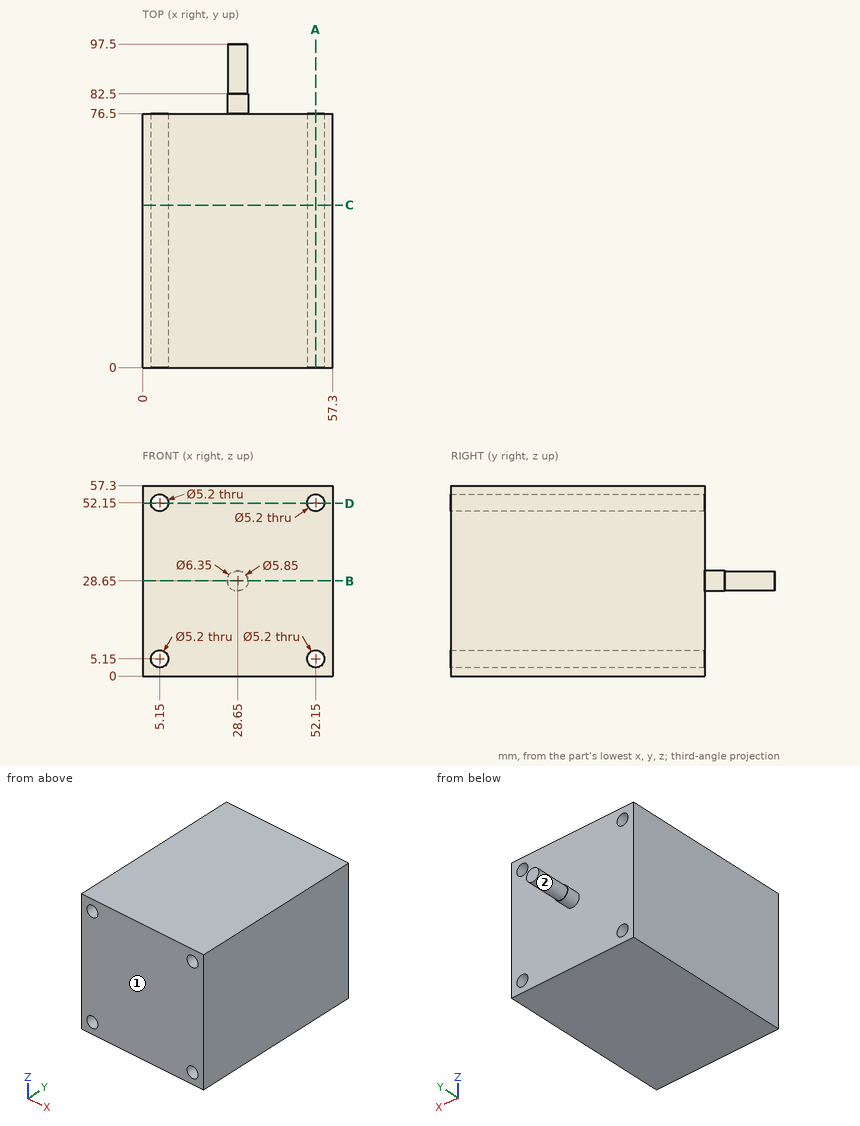
The figure shows three views and two pictorial views of one solid part (mm, origin at its lowest corner). Answer the questions. A direction names the side the tool comes from. Coordinates: 2 decimals unless noted, no trailing zeros. Loops run counter-clockwise (first coordinate to the right, second up) from the corner with the lowest first, then second, coordinate; pieces in that order, holes last. Notation, with made-up numbers: M -36.5,23 L -15.5,23 A10 ccw -15.5,40 Z; hole C 75.25,58.5 d11. An arc over 180 degrees is marked long. Answer as CSV lines item,"result". Start each with the question number.
(1) The part is cut by section D-D (z = 52). Give the vertices of the cut face in (x, y), and give its area (3 significant figures).
(2) The part is cut by section A-A (x = 52.15). Give the vertices of the cut face in (y, z).
(3) The part is cut by section B-B (z = 28.65). Give the vertices of the cut face in (x, y) (3 decimals).
(4) The part is cut by section C-C (y = 49). Give the vertices of the cut face in (x, z), and give its area (3 significant figures).
(5) Find the intervals of material crossed by L1, parallel to X at y = 51.5, z = 52.15; L2, parallel to Z at x = 4, y = 72, in increasing order. Write a range as [from, to].
(6) For the marked faces 1 and 2, determine the directions among +Z, -Z, +X, -X, +Y, -Y from which every point of the face is accessible in a straight line to the end or side of a thin tool.
(7) Given pin 1 (5 mm diameter, centred on x = 17, z = 17, fed in from -Y); pin 2 (4 mm diameter, centred on x = 33, z = 21.5, fed in from +Y), each flat-ended and moving along its own axis, determine where each tip first touches the part or whether it passes through.
Determined:
1,outline,"M 0,0 L 2.55,0 L 2.55,76.5 L 0,76.5 Z; M 7.75,0 L 49.55,0 L 49.55,76.5 L 7.75,76.5 Z; M 54.75,0 L 57.3,0 L 57.3,76.5 L 54.75,76.5 Z"
1,area,"3,590 mm2"
2,outline,"M 0,0 L 76.5,0 L 76.5,2.55 L 0,2.55 Z; M 0,7.75 L 76.5,7.75 L 76.5,49.55 L 0,49.55 Z; M 0,54.75 L 76.5,54.75 L 76.5,57.3 L 0,57.3 Z"
3,outline,"M 0,0 L 57.3,0 L 57.3,76.5 L 31.825,76.5 L 31.825,82.5 L 31.575,82.5 L 31.575,97.5 L 25.725,97.5 L 25.725,82.5 L 25.475,82.5 L 25.475,76.5 L 0,76.5 Z"
4,outline,"M 0,0 L 57.3,0 L 57.3,57.3 L 0,57.3 Z; hole C 5.15,5.15 d5.2; hole C 5.15,52.15 d5.2; hole C 52.15,5.15 d5.2; hole C 52.15,52.15 d5.2"
4,area,"3,200 mm2"
5,L1,"[0, 2.55], [7.75, 49.55], [54.75, 57.3]"
5,L2,"[0, 2.82], [7.48, 49.82], [54.48, 57.3]"
6,face 1,"+Z, -Z, +X, -X, -Y"
6,face 2,"+Y"
7,pin 1,"y = 0"
7,pin 2,"y = 76.5"
